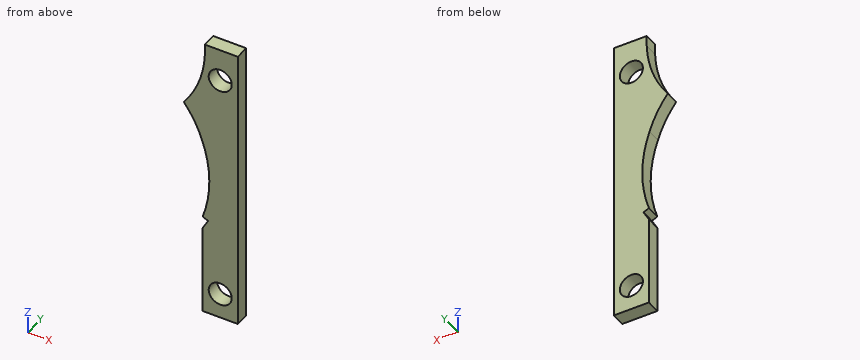
```python
from build123d import *

# Parameters (mm, degrees)
F0_R     = 5.2500022
F1_DEPTH = 6.35


# Not quite as in the source:
# - ends of sketch curves that miss each other by under 0.0002 mm in the source are joined


with BuildPart() as f1:
    # F0 (on Front) → F1 (new body)
    with BuildSketch(Plane.XZ):
        with BuildLine():
            Line((-2.7092148, 65.999995), (-2.7092148, 60.9999796))
            ThreePointArc((-2.7092148, 60.9999796), (-5.4016290161, 46.6516213468), (-12.2907672961, 33.7805612895))
            ThreePointArc((-12.2907672961, 33.7805612895), (-7.426360466, 26.392264731), (-3.9728687393, 18.248400136))
            ThreePointArc((-3.9728687393, 18.248400136), (-0.6755780926, -0.5535614771), (-3.7092166309, -19.3998583041))
            Line((-3.7092166309, -19.3998583041), (-1.2092178, -20.5000098))
            Line((-1.2092178, -20.5000098), (-3.7092128, -24.9706384))
            Line((-3.7092128, -24.9706384), (-3.7092128, -65.999995))
            Line((-3.7092128, -65.999995), (12.2907806, -65.999995))
            Line((12.2907806, -65.999995), (12.2907806, 65.999995))
            Line((12.2907806, 65.999995), (-2.7092148, 65.999995))
        make_face()
        with Locations((4.2907712, -54.4085272)):
            Circle(F0_R, mode=Mode.SUBTRACT)
        with Locations((4.2907712, 50.9999996)):
            Circle(F0_R, mode=Mode.SUBTRACT)
    extrude(amount=F1_DEPTH)


solid = f1.part
```
Check sheet for the modelled part. Datum: model origin and axes. Units: mm. Round coordinates to 2 decimals unless told otherwise and drop trailing zeros. Loops run counter-clockwise (first coordinate to the right, second up) from the corner with the lowest first, then second, coordinate; pieces in that order, holes last. Notation, with made-up numbers: (-4.5, 89) - (20.5, 89) arc R24 ccw to (20.5, 101) - close; hole circle Ø2 at (43, 55.25). An arc over 180 degrees is marked (long way). Answer as a JSON object with one key per item and string values. Group by question number.
Q1. Sectioned sample at A-A, the plane x = 4.75. Enter the section's corners in (y, z), plus the area to 3 significant figures.
Q2. Sectioned sample at C-C, the plane z = 51. Enter the section's corners in (x, y).
Q3. Scan lines: line 1 along Z through (x, y) = (0, -5); line 2 along Z through (x, y) = (2.5, -2); line 3 along X through (y, z) = (-3.25, 51). Record each from-to range of solid material in increasing order. Write a range as [from, to].
Q4. Gauge pin test, flat end, axial feed: P1, Ø8.5, axis at x = 4.29, z = 51, coming from the +Y side. Record the tip position at first contact, or that the pin passes through.
Q5. Sectioned sample at D-D, the plane z = 21. Enter the section's corners in (x, y).
Q6. Sectioned sample at B-B, the plane y = -3.25. Enter the section's corners in (x, z).
Solution:
{
 "1": {"outline": "(-6.35, -66) - (0, -66) - (0, -59.64) - (-6.35, -59.64) - close; (-6.35, -49.18) - (0, -49.18) - (0, 45.77) - (-6.35, 45.77) - close; (-6.35, 56.23) - (0, 56.23) - (0, 66) - (-6.35, 66) - close", "area": "705 mm²"},
 "2": {"outline": "(-4.1, -6.35) - (-0.96, -6.35) - (-0.96, 0) - (-4.1, 0) - close; (9.54, -6.35) - (12.29, -6.35) - (12.29, 0) - (9.54, 0) - close"},
 "3": {"line 1": "z = [-66, -57.43], [-51.38, 47.97], [54.03, 66]", "line 2": "z = [-66, -59.34], [-49.47, 46.06], [55.94, 66]", "line 3": "x = [-4.1, -0.96], [9.54, 12.29]"},
 "4": {"P1": "passes through"},
 "5": {"outline": "(-4.95, -6.35) - (12.29, -6.35) - (12.29, 0) - (-4.95, 0) - close"},
 "6": {"outline": "(-12.29, 33.78) arc R48.89 cw to (-3.97, 18.25) arc R57.56 cw to (-3.71, -19.4) - (-1.21, -20.5) - (-3.71, -24.97) - (-3.71, -66) - (12.29, -66) - (12.29, 66) - (-2.71, 66) - (-2.71, 61) arc R47.9 cw to start; hole circle Ø10.5 at (4.29, -54.41); hole circle Ø10.5 at (4.29, 51)"}
}
